from build123d import *

# Parameters (mm, degrees)
CROQUIS1_W              = 7
CROQUIS1_H              = 7
SALIENTE_EXTRUIR1_DEPTH = 6
CROQUIS2_R              = 0.25
SALIENTE_EXTRUIR2_DEPTH = 3
CROQUIS3_W              = 5
CROQUIS3_H              = 5
CORTAR_EXTRUIR1_DEPTH   = 1
CROQUIS4_W              = 0.5
CROQUIS4_H              = 1
CORTAR_EXTRUIR2_DEPTH   = 10


with BuildPart() as part:
    # Croquis1 → Saliente-Extruir1 (new body)
    with BuildSketch(Plane(origin=(0, 0, 0), x_dir=(1, 0, 0), z_dir=(0, 1, 0))):
        Rectangle(CROQUIS1_W, CROQUIS1_H)
    extrude(amount=SALIENTE_EXTRUIR1_DEPTH)

    # Croquis2 → Saliente-Extruir2 (add)
    with BuildSketch(Plane.XZ):
        with Locations((-1.27, 1.27)):
            Circle(CROQUIS2_R)
        with Locations((1.27, 1.27)):
            Circle(CROQUIS2_R)
        with Locations((1.27, -1.27)):
            Circle(CROQUIS2_R)
        with Locations((-1.27, -1.27)):
            Circle(CROQUIS2_R)
    extrude(amount=SALIENTE_EXTRUIR2_DEPTH)

    # Croquis3 → Cortar-Extruir1 (cut)
    with BuildSketch(Plane(origin=(0, 6, 0), x_dir=(1, 0, 0), z_dir=(0, 1, 0))):
        Rectangle(CROQUIS3_W, CROQUIS3_H)
    extrude(amount=-CORTAR_EXTRUIR1_DEPTH, mode=Mode.SUBTRACT)

    # Croquis4 → Cortar-Extruir2 (cut, through all)
    with BuildSketch(Plane(origin=(0, 6, 0), x_dir=(1, 0, 0), z_dir=(0, 1, 0))):
        with Locations((3.5, 0)):
            Rectangle(CROQUIS4_W, CROQUIS4_H)
        with Locations((-3.5, 0)):
            Rectangle(CROQUIS4_W, CROQUIS4_H)
    extrude(amount=-CORTAR_EXTRUIR2_DEPTH, mode=Mode.SUBTRACT)


solid = part.part
Verification items for the finished model (mm, model axes). A direction names the side the tool comes from. Coordinates: 2 decimals unless noted, no trailing zeros. Order: outer loops, then holes, each group sorted by start corner. A loop starts at its lowest first (then second) coordinate and runs counter-clockwise, first axis right, second up.
1. Release check for a two-part mould opening along Z. For faces 4 (the face through (-3.5, 3, -2)), 5 (the face through (0, 3, -3.5)), 6 (the face through (3.25, 3, 0)) record: +Z half, -Z half, draft (parallel to the pull), parting line (faces both ways), or undercut.
Results found:
face 4: draft
face 5: -Z half
face 6: undercut
2. Sectioned sample at B-B, the plane z = -1.27. Record the cut outline in (x, y).
Results found:
outline: (-3.5, 0) - (-1.52, 0) - (-1.52, -3) - (-1.02, -3) - (-1.02, 0) - (1.02, 0) - (1.02, -3) - (1.52, -3) - (1.52, 0) - (3.5, 0) - (3.5, 6) - (2.5, 6) - (2.5, 5) - (-2.5, 5) - (-2.5, 6) - (-3.5, 6) - close
3. Sectioned sample at C-C, the plane y = -1. Record the cut outline in (x, z), and give its area (3 significant figures).
Results found:
outline: circle Ø0.5 at (-1.27, -1.27); circle Ø0.5 at (-1.27, 1.27); circle Ø0.5 at (1.27, -1.27); circle Ø0.5 at (1.27, 1.27)
area: 0.785 mm2
4. Sectioned sample at A-A, the plane x = -1.27. Record the cut outline in (y, z), and give its area (3 significant figures).
Results found:
outline: (-3, -1.52) - (0, -1.52) - (0, -3.5) - (6, -3.5) - (6, -2.5) - (5, -2.5) - (5, 2.5) - (6, 2.5) - (6, 3.5) - (0, 3.5) - (0, 1.52) - (-3, 1.52) - (-3, 1.02) - (0, 1.02) - (0, -1.02) - (-3, -1.02) - close
area: 40.0 mm2
5. Set-up check for faces 1 (the face through (3.5, 3, 2)), 2 (the face through (2.5, 5.5, 0)), 3 (the face through (-3.25, 3, 0)): record each of +Z, -Z, +X, -X, +Y, -Y from which the full face is reachable in a straight line by a thin tool's end or side.
Results found:
face 1: +Z, -Z, +X, +Y, -Y
face 2: +Y
face 3: -X, +Y, -Y
6. Sectioned sample at D-D, the plane x = 0.25. Record the cut outline in (y, z).
Results found:
outline: (0, -3.5) - (6, -3.5) - (6, -2.5) - (5, -2.5) - (5, 2.5) - (6, 2.5) - (6, 3.5) - (0, 3.5) - close
7. Scan lines: line 1 (Y direction, x = -1.25, z = 3.25); line 2 (X direction, y = -1, z = 1.25); line 3 (Y direction, x = 0, z = -1.5). Record each from-to range of solid material in increasing order.
Results found:
line 1: y = 0 to 6
line 2: x = -1.52 to -1.02, 1.02 to 1.52
line 3: y = 0 to 5
8. Go/stop test with flat-tipped pins: pin 1 Ø0.5 at (y, z) = (5.5, 0) entering from -X; pin 2 Ø1.5 at (x, z) = (1, -1) entering from +Y. Record where each tip stops, or that it passes through.
Results found:
pin 1: stops at x = -3.25
pin 2: stops at y = 5
